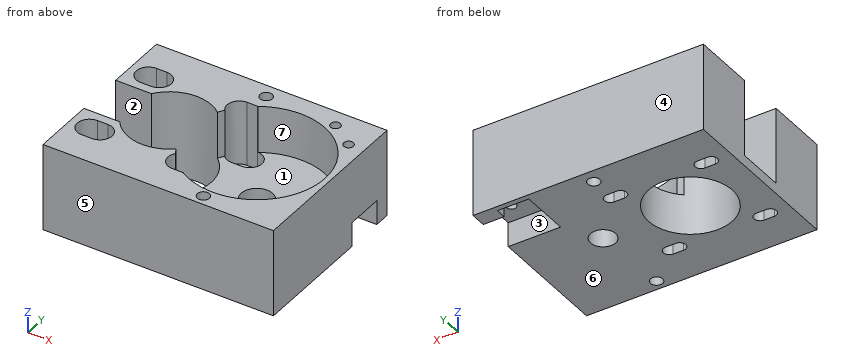
from build123d import *

# Parameters (mm, degrees)
BOX043_W          = 20
BOX043_H          = 14
BOX043_DEPTH      = 30
CYLINDER032_R     = 1.75
CYLINDER032_DEPTH = 200
CYLINDER031_R     = 1.75
CYLINDER031_DEPTH = 200
CYLINDER072_R     = 1.4
CYLINDER072_DEPTH = 50
CYLINDER071_R     = 1.4
CYLINDER071_DEPTH = 50
BOX042_W          = 9
BOX042_H          = 5
BOX042_DEPTH      = 7
BOX040_W          = 50
BOX040_H          = 11
BOX040_DEPTH      = 7
CYLINDER019_R     = 4.5
CYLINDER019_DEPTH = 30
CYLINDER018_R     = 3.6
CYLINDER018_DEPTH = 30
CYLINDER016_R     = 19.5
CYLINDER016_DEPTH = 20
CYLINDER017_R     = 12
CYLINDER017_DEPTH = 33
BOX003_W          = 3
BOX003_H          = 7
BOX003_DEPTH      = 25
CYLINDER020_R     = 1.7
CYLINDER020_DEPTH = 25
CYLINDER012_R     = 3.5
CYLINDER012_DEPTH = 25
BOX002_W          = 3
BOX002_H          = 3.4
BOX002_DEPTH      = 15
CYLINDER021_R     = 3.5
CYLINDER021_DEPTH = 25
CYLINDER008_R     = 1.7
CYLINDER008_DEPTH = 25
BOX001_W          = 66
BOX001_H          = 50
BOX001_DEPTH      = 25


with BuildPart() as cube040:
    # Box043 → Box043 (new body)
    with BuildSketch(Plane(origin=(-21, -7, 29), x_dir=(1, 0, 0), z_dir=(0, 0, 1))):
        with Locations((10, 7)):
            Rectangle(BOX043_W, BOX043_H)
    extrude(amount=BOX043_DEPTH)


with BuildPart() as m3_studding003:
    # Cylinder032 → Cylinder032 (new body)
    with BuildSketch(Plane(origin=(24, -22, 0), x_dir=(1, 0, 0), z_dir=(0, 0, 1))):
        Circle(CYLINDER032_R)
    extrude(amount=CYLINDER032_DEPTH)


with BuildPart() as long_stack_studding_a:
    # Cylinder031 → Cylinder031 (new body)
    with BuildSketch(Plane(origin=(14, 21, 0), x_dir=(1, 0, 0), z_dir=(0, 0, 1))):
        Circle(CYLINDER031_R)
    extrude(amount=CYLINDER031_DEPTH)

    # Fusion046: union m3-studding003
    add(m3_studding003.part)


with BuildPart() as m3_studding013:
    # Cylinder072 → Cylinder072 (new body)
    with BuildSketch(Plane(origin=(41.5, 15, -6), x_dir=(1, 0, 0), z_dir=(0, 0, 1))):
        Circle(CYLINDER072_R)
    extrude(amount=CYLINDER072_DEPTH)


with BuildPart() as m3_tap001:
    # Cylinder071 → Cylinder071 (new body)
    with BuildSketch(Plane(origin=(34.5, 20, -6), x_dir=(1, 0, 0), z_dir=(0, 0, 1))):
        Circle(CYLINDER071_R)
    extrude(amount=CYLINDER071_DEPTH)

    # Fusion042: union m3-studding013
    add(m3_studding013.part)


with BuildPart() as m3_tap001_1:
    # Fusion042 placement: moved
    add(m3_tap001.part.moved(Location((0, 0, 10))))


with BuildPart() as cube039:
    # Box042 → Box042 (new body)
    with BuildSketch(Plane(origin=(31, 18.5, 26), x_dir=(1, 0, 0), z_dir=(0, 0, 1))):
        with Locations((4.5, 2.5)):
            Rectangle(BOX042_W, BOX042_H)
    extrude(amount=BOX042_DEPTH)


with BuildPart() as cube037:
    # Box040 → Box040 (new body)
    with BuildSketch(Plane(origin=(31, 9.5, 26), x_dir=(1, 0, 0), z_dir=(0, 0, 1))):
        with Locations((25, 5.5)):
            Rectangle(BOX040_W, BOX040_H)
    extrude(amount=BOX040_DEPTH)


with BuildPart() as f_9mm_bearing:
    # Cylinder019 → Cylinder019 (new body)
    with BuildSketch(Plane(origin=(25, 0, 32.5), x_dir=(1, 0, 0), z_dir=(0, 0, 1))):
        Circle(CYLINDER019_R)
    extrude(amount=CYLINDER019_DEPTH)


with BuildPart() as bearing_and_shaft_holes:
    # Cylinder018 → Cylinder018 (new body)
    with BuildSketch(Plane(origin=(25, 0, 24), x_dir=(1, 0, 0), z_dir=(0, 0, 1))):
        Circle(CYLINDER018_R)
    extrude(amount=CYLINDER018_DEPTH)

    # Fusion007: union 9mm-bearing
    add(f_9mm_bearing.part)


with BuildPart() as big_gear_hole:
    # Cylinder016 → Cylinder016 (new body)
    with BuildSketch(Plane(origin=(25, 0, 37.5), x_dir=(1, 0, 0), z_dir=(0, 0, 1))):
        Circle(CYLINDER016_R)
    extrude(amount=CYLINDER016_DEPTH)


with BuildPart() as gear_holes:
    # Cylinder017 → Cylinder017 (new body)
    with BuildSketch(Plane.XY.offset(25)):
        Circle(CYLINDER017_R)
    extrude(amount=CYLINDER017_DEPTH)

    # Fusion006: union big-gear-hole
    add(big_gear_hole.part)


with BuildPart() as cube003:
    # Box003 → Box003 (new body)
    with BuildSketch(Plane(origin=(13, 9.5, 35.5), x_dir=(1, 0, 0), z_dir=(0, 0, 1))):
        with Locations((1.5, 3.5)):
            Rectangle(BOX003_W, BOX003_H)
    extrude(amount=BOX003_DEPTH)


with BuildPart() as cylinder020:
    # Cylinder020 → Cylinder020 (new body)
    with BuildSketch(Plane(origin=(16, 13, 25), x_dir=(1, 0, 0), z_dir=(0, 0, 1))):
        Circle(CYLINDER020_R)
    extrude(amount=CYLINDER020_DEPTH)


with BuildPart() as cylinder012:
    # Cylinder012 → Cylinder012 (new body)
    with BuildSketch(Plane(origin=(13, 13, 35.5), x_dir=(1, 0, 0), z_dir=(0, 0, 1))):
        Circle(CYLINDER012_R)
    extrude(amount=CYLINDER012_DEPTH)


with BuildPart() as cube002:
    # Box002 → Box002 (new body)
    with BuildSketch(Plane(origin=(13, 11.3, 25), x_dir=(1, 0, 0), z_dir=(0, 0, 1))):
        with Locations((1.5, 1.7)):
            Rectangle(BOX002_W, BOX002_H)
    extrude(amount=BOX002_DEPTH)


with BuildPart() as cylinder021:
    # Cylinder021 → Cylinder021 (new body)
    with BuildSketch(Plane(origin=(16, 13, 35.5), x_dir=(1, 0, 0), z_dir=(0, 0, 1))):
        Circle(CYLINDER021_R)
    extrude(amount=CYLINDER021_DEPTH)


with BuildPart() as cylinder008:
    # Cylinder008 → Cylinder008 (new body)
    with BuildSketch(Plane(origin=(13, 13, 25), x_dir=(1, 0, 0), z_dir=(0, 0, 1))):
        Circle(CYLINDER008_R)
    extrude(amount=CYLINDER008_DEPTH)


with BuildPart() as m3_slot001:
    # Fusion002 base: copy of Cylinder008
    add(cylinder008.part)

    # Fusion002: union Cube003, Cylinder020, Cylinder012, Cube002, Cylinder021
    add(cube003.part)
    add(cylinder020.part)
    add(cylinder012.part)
    add(cube002.part)
    add(cylinder021.part)


with BuildPart() as m3_slot001_1:
    # Fusion002 placement: moved
    add(m3_slot001.part.moved(Location((-27.5, 0, 0))))


with BuildPart() as m3_slot002:
    # Fusion003 base: copy of Cylinder008
    add(cylinder008.part)

    # Fusion003: union Cube003, Cylinder020, Cylinder012, Cube002, Cylinder021
    add(cube003.part)
    add(cylinder020.part)
    add(cylinder012.part)
    add(cube002.part)
    add(cylinder021.part)


with BuildPart() as m3_slot002_1:
    # Fusion003 placement: moved
    add(m3_slot002.part.moved(Location((-27.5, -26, 0))))


with BuildPart() as m3_slot003:
    # Fusion004 base: copy of Cylinder008
    add(cylinder008.part)

    # Fusion004: union Cube003, Cylinder020, Cylinder012, Cube002, Cylinder021
    add(cube003.part)
    add(cylinder020.part)
    add(cylinder012.part)
    add(cube002.part)
    add(cylinder021.part)


with BuildPart() as m3_slot003_1:
    # Fusion004 placement: moved
    add(m3_slot003.part.moved(Location((-1.5, -26, 0))))


with BuildPart() as fusion008:
    # Fusion001 base: copy of Cylinder008
    add(cylinder008.part)

    # Fusion001: union Cube003, Cylinder020, Cylinder012, Cube002, Cylinder021
    add(cube003.part)
    add(cylinder020.part)
    add(cylinder012.part)
    add(cube002.part)
    add(cylinder021.part)


with BuildPart() as fusion008_1:
    # Fusion001 placement: moved
    add(fusion008.part.moved(Location((-1.5, 0, 0))))

    # Fusion005: union M3-slot001, M3-slot002, M3-slot003
    add(m3_slot001_1.part)
    add(m3_slot002_1.part)
    add(m3_slot003_1.part)


with BuildPart() as fusion008_2:
    # Fusion005 placement: moved
    add(fusion008_1.part.moved(Location((0, 0, -3))))

    # Fusion008: union bearing-and-shaft-holes, gear-holes
    add(bearing_and_shaft_holes.part)
    add(gear_holes.part)


with BuildPart() as gearbox:
    # Box001 → Box001 (new body)
    with BuildSketch(Plane(origin=(-20, -25, 26), x_dir=(1, 0, 0), z_dir=(0, 0, 1))):
        with Locations((33, 25)):
            Rectangle(BOX001_W, BOX001_H)
    extrude(amount=BOX001_DEPTH)

    # Cut: cut Fusion008
    add(fusion008_2.part, mode=Mode.SUBTRACT)

    # Cut023: cut Cube037
    add(cube037.part, mode=Mode.SUBTRACT)

    # Cut028: cut Cube039
    add(cube039.part, mode=Mode.SUBTRACT)

    # Cut030: cut M3-tap001
    add(m3_tap001_1.part, mode=Mode.SUBTRACT)

    # Cut034: cut long-stack-studding-a
    add(long_stack_studding_a.part, mode=Mode.SUBTRACT)

    # Cut041: cut Cube040
    add(cube040.part, mode=Mode.SUBTRACT)


solid = gearbox.part
Part model, mm, in its own coordinate system. Face numbers are marked on the shaded views. A direction names the side the tool comes from. Give positions to 0.01 mm unless a question says otherwise; leave off trailing zeros. Write each loop counter-clockwise with the first axis right and the second up, starting at its lowest first coordinate (ties: lowest second). Pieces come first, ordered by that corner, then holes.
1) Two-plate mould, pull along Y, no slides. Class the marked faces 4, 5, 6 and 7: released by +Y, released by -Y, zero draft, split by the parting line, or undercut.
Resolved:
face 4: released by +Y
face 5: released by -Y
face 6: zero draft
face 7: undercut
2) Cut at A-A on z = 31.5. State how many separate pieces and enclosed holes the cut face has, then the cut area to 3 significant figures.
Resolved:
separate pieces: 1
enclosed holes: 7
area: 2,400 mm2
3) Cut at C-C on y = -13. Write the cut outline in (x, z).
Resolved:
outline: (-20, 26) - (-16.2, 26) - (-16.2, 32.5) - (-18, 32.5) - (-18, 51) - (-20, 51) - close; (-9.8, 26) - (9.8, 26) - (9.8, 32.5) - (8, 32.5) - (8, 51) - (-8, 51) - (-8, 32.5) - (-9.8, 32.5) - close; (16.2, 26) - (46, 26) - (46, 51) - (39.53, 51) - (39.53, 37.5) - (18, 37.5) - (18, 32.5) - (16.2, 32.5) - close
4) Which spindle directions (+Z, -Z, +X, -X, +Y, -Y) get a long thin tool onto all of the face, cutting with end or side? Do the marked faces 1, 2 and 3. Say none if no direction does.
Resolved:
face 1: +Z
face 2: +Z, -X
face 3: -Z, +X
5) Cut at B-B on x = 25. Write the cut outline in (y, z).
Resolved:
outline: (-25, 26) - (-23.44, 26) - (-23.44, 51) - (-25, 51) - close; (-20.56, 26) - (-3.6, 26) - (-3.6, 32.5) - (-4.5, 32.5) - (-4.5, 37.5) - (-19.5, 37.5) - (-19.5, 51) - (-20.56, 51) - close; (3.6, 26) - (25, 26) - (25, 51) - (19.5, 51) - (19.5, 37.5) - (4.5, 37.5) - (4.5, 32.5) - (3.6, 32.5) - close
6) Cut at D-D on x = 41.5. Write the cut outline in (y, z), then the cut area to 3 significant figures.
Resolved:
outline: (-25, 26) - (9.5, 26) - (9.5, 33) - (13.6, 33) - (13.6, 51) - (10.39, 51) - (10.39, 37.5) - (-10.39, 37.5) - (-10.39, 51) - (-25, 51) - close; (16.4, 33) - (20.5, 33) - (20.5, 26) - (25, 26) - (25, 51) - (16.4, 51) - close
area: 842 mm2
7) Probe L1, parallel to X at y = 21, z = 32.5; L2, parallel to X at y = -22, z = 27; L3, parallel to Y at x = 14.5, z = 46.75. List the from-to ranges inside material, lowest first.
Resolved:
L1: x = -20 to 12.25, 15.75 to 31, 40 to 46
L2: x = -20 to 22.25, 25.75 to 46
L3: y = -25 to -16.5, 16.5 to 19.32, 22.68 to 25
8) Pin check, flat tips, straight feed: pin 1 (2 mm diameter, centred on x = 14, y = 21, fed in from +Z); pin 2 (2 mm diameter, centred on x = 14, y = 11.5, fed in from +Z); pin 3 (7 mm diameter, centred on x = 26, y = -2, fed in from +Z). Stop position of each tip, or through.
Resolved:
pin 1: passes through
pin 2: stops at z = 32.5
pin 3: stops at z = 37.5
